The model under review builds one solid part; all positions refer to its coordinate system, in mm. A direction names the side the tool comes from. Round coordinates to 2 decimals unless told otherwise and drop trailing zeros. Write each loop counter-clockwise with the first axis right and the second up, starting at its lowest first coordinate (ties: lowest second). Pieces come first, ordered by that corner, then holes. Notation, with made-up numbers: M 7.25,44 L 50.25,44 A17 cw 50.25,57 Z; hole C 78.25,9 d5. An arc over 180 degrees is marked long. Write item = value, one per line. Start each with the question number.
Item 1: Tool access review of faces 1 (the cylindrical face through (58.35, 0.07, 1.97)), 2 (the flat face through (30, 0, 25)): name each direction out of +Z, -Z, +X, -X, +Y, -Y from which nothing blocks a thin tool from reaching the whole face with its end or side.
Item 2: To check wall thickness, follow line 1 along Z through (x, y) = (26.5, 0.2); line 2 along Z through (x, y) = (37.5, 1.9); line 3 along X through (y, z) = (0, 17). State the ranges of each line that lie inside material, in increasing order.
Item 3: Take a section at A-A, the plane x = 21.5. Give the boundary of the cut face in (y, z).
Item 4: The part is to be moulded in two halves that separate along X. For faces 3 (the cylindrical face through (63, 0, 2)), 4 (the flat face through (24, 0, 19)), 5 (the flat face through (30, 0, 58)), 6 (the cylindrical face through (17.1, -0.03, 44.43)), say which applies: +X half, -X half, draft (parallel to the pull), parting line (faces both ways), or undercut.
Item 5: Take a section at C-C, the plane z = 41.5. Give the boundary of the cut face in (x, y), plus the area to 3 significant figures.
Item 6: Take a section at D-D, the plane z = 7. Give the boundary of the cut face in (x, y).
Item 7: For pin 1 Ø1 at (y, z) = (2.5, 44.5) entering from +X, flat-tipped, find the tip position at first contact; note if it passes through.
Item 8: Take a section at B-B, the plane y = 0. Give the number of separate pieces and of enclosed holes in the cut face, plus the area to 3 significant figures.
from build123d import *

# Parameters (mm, degrees)
SKETCH1_R           = 1.65
BOSS_EXTRUDE1_DEPTH = 4
BOSS_EXTRUDE2_DEPTH = 25
CUT_EXTRUDE1_DEPTH  = 25
FILLET1_R           = 1


with BuildPart() as part:
    # Sketch1 → Boss-Extrude1 (new body)
    with BuildSketch(Plane.XY):
        with BuildLine():
            ThreePointArc((0, 3), (-3, 0), (0, -3))
            Line((0, -3), (60, -3))
            ThreePointArc((60, -3), (63, 0), (60, 3))
            Line((60, 3), (0, 3))
        make_face()
        Circle(SKETCH1_R, mode=Mode.SUBTRACT)
        with Locations((60, 0)):
            Circle(SKETCH1_R, mode=Mode.SUBTRACT)
    extrude(amount=BOSS_EXTRUDE1_DEPTH)

    # Sketch2 → Boss-Extrude2 (add)
    with BuildSketch(Plane.XY.offset(4)):
        Polygon((55, -2.5), (5, 2.5), (5, -3), (55, -3), align=None)
        Polygon((5, 3), (5, 2.5), (55, -2.5), (55, 3), align=None)
    extrude(amount=BOSS_EXTRUDE2_DEPTH)

    # Mirror1: part across plane


with BuildPart() as part_1:
    add(part.part)
    add(part.part.mirror(Plane.XY.offset(29)))

    # Sketch4 → Cut-Extrude1 (cut)
    with BuildSketch(Plane.XZ.offset(3)):
        with BuildLine():
            Line((16.5, 42.5), (26, 33))
            Line((26, 33), (41.5, 33))
            ThreePointArc((41.5, 33), (42.914213562, 33.585786438), (43.5, 35))
            Line((43.5, 35), (43.5, 43))
            ThreePointArc((43.5, 43), (42.914213562, 44.414213562), (41.5, 45))
            Line((41.5, 45), (18.5, 45))
            ThreePointArc((18.5, 45), (17.085786438, 44.414213562), (16.5, 43))
            Line((16.5, 43), (16.5, 42.5))
        make_face()
        with BuildLine():
            Line((18.5, 33), (26, 33))
            Line((26, 33), (16.5, 42.5))
            Line((16.5, 42.5), (16.5, 35))
            ThreePointArc((16.5, 35), (17.085786438, 33.585786438), (18.5, 33))
        make_face()
        with BuildLine():
            Line((36, 23), (34, 25))
            Line((34, 25), (26, 25))
            ThreePointArc((26, 25), (24.585786438, 24.414213562), (24, 23))
            Line((24, 23), (24, 15))
            ThreePointArc((24, 15), (24.585786438, 13.585786438), (26, 13))
            Line((26, 13), (34, 13))
            ThreePointArc((34, 13), (35.414213562, 13.585786438), (36, 15))
            Line((36, 15), (36, 23))
        make_face()
        with BuildLine():
            ThreePointArc((36, 23), (35.414213562, 24.414213562), (34, 25))
            Line((34, 25), (36, 23))
        make_face()
    extrude(amount=-CUT_EXTRUDE1_DEPTH, mode=Mode.SUBTRACT)

    # Fillet1
    fillet1_edges = [part_1.edges().sort_by_distance(p)[0] for p in [
        (24.585786438, -3, 13.585786438),
        (30, -3, 25),
        (36, -3, 19),
        (30, -3, 13),
        (35.414213562, -3, 13.585786438),
        (35.414213562, -3, 24.414213562),
        (24.585786438, -3, 24.414213562),
        (24, -3, 19),
        (55, -3, 29),
        (55, 3, 29),
        (5, 3, 29),
        (5, -3, 29),
        (30, 3, 13),
        (35.414213562, 3, 13.585786438),
        (36, 3, 19),
        (35.414213562, 3, 24.414213562),
        (30, 3, 25),
        (24.585786438, 3, 24.414213562),
        (24, 3, 19),
        (24.585786438, 3, 13.585786438),
        (17.085786438, 3, 44.414213562),
        (16.5, 3, 39),
        (17.085786438, 3, 33.585786438),
        (30, 3, 33),
        (42.914213562, 3, 33.585786438),
        (43.5, 3, 39),
        (42.914213562, 3, 44.414213562),
        (30, 3, 45),
        (30, -3, 45),
        (43.5, -3, 39),
        (42.914213562, -3, 33.585786438),
        (17.085786438, -3, 33.585786438),
        (17.085786438, -3, 44.414213562),
        (16.5, -3, 39),
        (30, -3, 33),
        (42.914213562, -3, 44.414213562),
    ]]
    fillet(fillet1_edges, radius=FILLET1_R)


solid = part_1.part
Response values:
q1.face_1 = +Z, -Z
q1.face_2 = +Y, -Y
q2.line_1 = 0 to 13, 25 to 33, 45 to 58
q2.line_2 = 0 to 33, 45 to 58
q2.line_3 = 5 to 24, 36 to 55
q3.outline = M -3,0 L 3,0 L 3,32 A1 ccw 2,33 L -2,33 A1 ccw -3,32 Z; M -3,46 A1 ccw -2,45 L 2,45 A1 ccw 3,46 L 3,58 L -3,58 Z
q4.face_3 = +X half
q4.face_4 = undercut
q4.face_5 = draft
q4.face_6 = undercut
q5.outline = M 5,-2 A1 ccw 6,-3 L 15.5,-3 A1 ccw 16.5,-2 L 16.5,2 A1 ccw 15.5,3 L 6,3 A1 ccw 5,2 Z; M 43.5,-2 A1 ccw 44.5,-3 L 54,-3 A1 ccw 55,-2 L 55,2 A1 ccw 54,3 L 44.5,3 A1 ccw 43.5,2 Z
q5.area = 136 mm2
q6.outline = M 5,-2 A1 ccw 6,-3 L 54,-3 A1 ccw 55,-2 L 55,2 A1 ccw 54,3 L 6,3 A1 ccw 5,2 Z
q7.pin_1 = 55
q8.separate_pieces = 5
q8.enclosed_holes = 2
q8.area = 2,510 mm2
